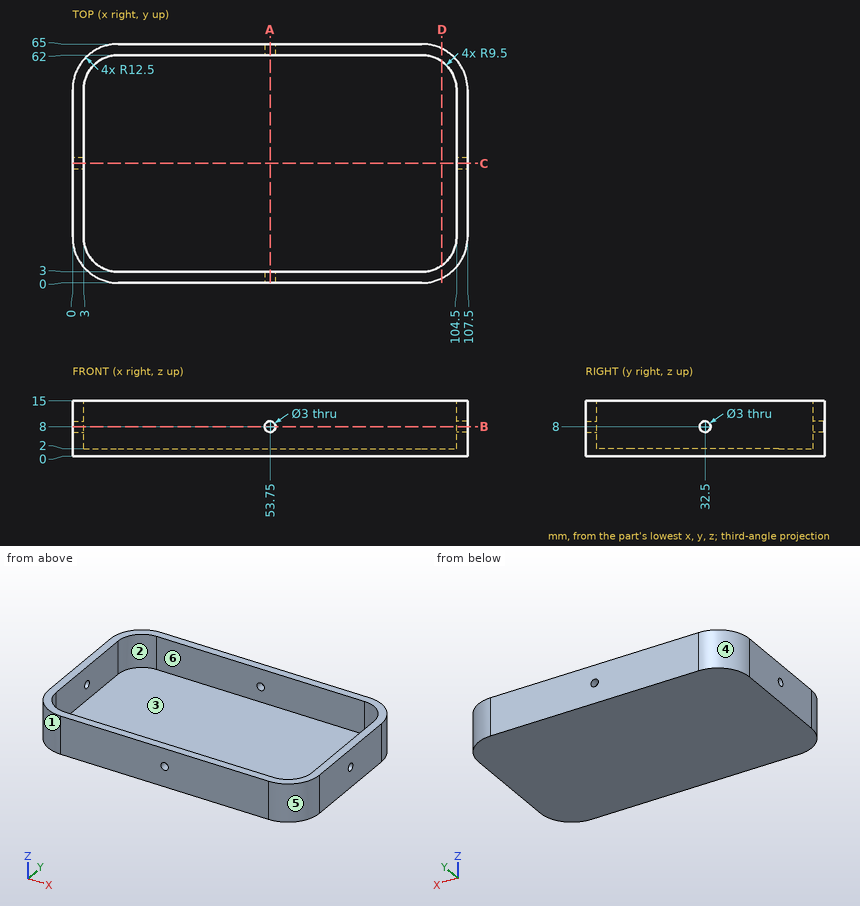
Could you check a few things on this drawing? It's one solid part, dimensions in mm from its lowest x, y, z. A direction names the side the tool comes from. Coordinates: 2 decimals unless noted, no trailing zeros. Loops run counter-clockwise (first coordinate to the right, second up) from the corner with the lowest first, then second, coordinate; pieces in that order, holes last. Notation, with made-up numbers: (-11.5, 69.25) - (-5.5, 69.25) arc R17 cw to (-5.5, 73.25) - close; hole circle Ø6 at (22.25, 35). An arc over 180 degrees is marked (long way). Return JSON: item names as keys, results as strings. Group by question number.
Item 1: Will these pins go through, and if not, where does the flat tip stop? P1, Ø1.8, axis at y = 32.5, z = 8, coming from the -X side; P2, Ø1, axis at y = 8, z = 12.5, coming from the -X side.
Item 2: On a 3-axis mill with a long thin cutter (end or side, diameter ignored), from which of +Z, -Z, +X, -X, +Y, -Y can I reach the whole of each face in a straight line? I mean the marked faces 5 and 6. Say none if no direction works.
Item 3: We'd pull the mould along Y, two halves only. Please class the marked faces 1, 2, 3 and 4: +Y half, -Y half, draft (parallel to the pull), parting line (faces both ways), or undercut.
Item 4: If we section it at D-D on x = 100.5: Write out the boundary of the cut face in (y, z).
Item 5: If we section it at C-C on y = 32.5: Write out the boundary of the cut face in (x, z).
Item 6: If we section it at B-B on z = 8: State how many separate pieces and enclosed holes the cut face has, and give its area (3 significant figures).
Item 7: If we section it at A-A on x = 53.75: Write out the boundary of the cut face in (y, z).
Item 8: I need wall thicknesses on line 1 (Y direction, x = 89.5, z = 10.25); line 2 (X direction, y = 16, z = 5); line 3 (Z direction, x = 41.5, y = 51). Which ranges of each line are inside material? Lowest first, please. Write a range as from..to.
Calculated:
{
 "1": {"P1": "passes through", "P2": "stops at x = 0.66"},
 "2": {"face 5": "+Z, -Z, +X, -Y", "face 6": "+Z"},
 "3": {"face 1": "-Y half", "face 2": "undercut", "face 3": "undercut", "face 4": "+Y half"},
 "4": {"outline": "(1.28, 0) - (63.72, 0) - (63.72, 15) - (60.25, 15) - (60.25, 2) - (4.75, 2) - (4.75, 15) - (1.28, 15) - close"},
 "5": {"outline": "(0, 0) - (107.5, 0) - (107.5, 6.5) - (104.5, 6.5) - (104.5, 2) - (3, 2) - (3, 6.5) - (0, 6.5) - close; (0, 9.5) - (3, 9.5) - (3, 15) - (0, 15) - close; (104.5, 9.5) - (107.5, 9.5) - (107.5, 15) - (104.5, 15) - close"},
 "6": {"separate pieces": "4", "enclosed holes": "0", "area": "906 mm^2"},
 "7": {"outline": "(0, 0) - (65, 0) - (65, 6.5) - (62, 6.5) - (62, 2) - (3, 2) - (3, 6.5) - (0, 6.5) - close; (0, 9.5) - (3, 9.5) - (3, 15) - (0, 15) - close; (62, 9.5) - (65, 9.5) - (65, 15) - (62, 15) - close"},
 "8": {"line 1": "y = 0..3, 62..65", "line 2": "x = 0..3, 104.5..107.5", "line 3": "z = 0..2"}
}
